The listing builds one solid part. Answer for the finished solid, in the listing's coordinates (mm). A direction names the side the tool comes from. Give positions to 0.01 mm unless a question says otherwise; leave off trailing zeros. Write each loop counter-clockwise with the first axis right and the second up, starting at its lowest first coordinate (ties: lowest second). Pieces come first, ordered by that corner, then holes. Notation, with made-up numbers: M 25.5,-5 L 72.5,-5 A18 ccw 72.5,21 Z; hole C 24,34 d1. An arc over 180 degrees is marked long. Answer as a JSON object with one key per item and string values.
```python
from build123d import *

# Parameters (mm, degrees)
SKETCH1_R           = 3.3274
BOSS_EXTRUDE1_DEPTH = 100


with BuildPart() as part:
    # Sketch1 → Boss-Extrude1 (new, symmetric)
    with BuildSketch(Plane.XY):
        with BuildLine():
            Line((-10.287, 13.552357131), (-10.287, 14.0843))
            ThreePointArc((-10.287, 14.0843), (-10.022898185, 14.721898185), (-9.3853, 14.986))
            Line((-9.3853, 14.986), (-5.617617549, 14.986))
            ThreePointArc((-5.617617549, 14.986), (-4.519044045, 15.441044045), (-4.064, 16.539617549))
            Line((-4.064, 16.539617549), (-4.064, 17.496382451))
            ThreePointArc((-4.064, 17.496382451), (-4.519044045, 18.594955955), (-5.617617549, 19.05))
            Line((-5.617617549, 19.05), (-7.974178704, 19.05))
            Line((-7.974178704, 19.05), (-15.847487039, 19.05))
            ThreePointArc((-15.847487039, 19.05), (-18.120176289, 18.120192083), (-19.05, 15.847509295))
            Line((-19.05, 15.847509295), (-19.05, 7.97632366))
            Line((-19.05, 7.97632366), (-19.05, 5.617617549))
            ThreePointArc((-19.05, 5.617617549), (-18.594955955, 4.519044045), (-17.496382451, 4.064))
            Line((-17.496382451, 4.064), (-16.539617549, 4.064))
            ThreePointArc((-16.539617549, 4.064), (-15.441044045, 4.519044045), (-14.986, 5.617617549))
            Line((-14.986, 5.617617549), (-14.986, 9.385342516))
            ThreePointArc((-14.986, 9.385342516), (-14.721898185, 10.022940701), (-14.0843, 10.287042516))
            Line((-14.0843, 10.287042516), (-13.516042086, 10.287042516))
            ThreePointArc((-13.516042086, 10.287042516), (-13.170975923, 10.218404478), (-12.878443117, 10.022939917))
            Line((-12.878443117, 10.022939917), (-8.14758008, 5.292065243))
            ThreePointArc((-8.14758008, 5.292065243), (-7.117955879, 3.751120653), (-6.7564, 1.933453584))
            Line((-6.7564, 1.933453584), (-6.7564, -1.933453584))
            ThreePointArc((-6.7564, -1.933453584), (-7.117955879, -3.751120653), (-8.14758008, -5.292065243))
            Line((-8.14758008, -5.292065243), (-12.878443117, -10.022939917))
            ThreePointArc((-12.878443117, -10.022939917), (-13.170975923, -10.218404478), (-13.516042086, -10.287042516))
            Line((-13.516042086, -10.287042516), (-14.0843, -10.287042516))
            ThreePointArc((-14.0843, -10.287042516), (-14.721898185, -10.022940701), (-14.986, -9.385342516))
            Line((-14.986, -9.385342516), (-14.986, -5.617617549))
            ThreePointArc((-14.986, -5.617617549), (-15.441044045, -4.519044045), (-16.539617549, -4.064))
            Line((-16.539617549, -4.064), (-17.496382451, -4.064))
            ThreePointArc((-17.496382451, -4.064), (-18.594955955, -4.519044045), (-19.05, -5.617617549))
            Line((-19.05, -5.617617549), (-19.05, -7.976318491))
            Line((-19.05, -7.976318491), (-19.05, -15.847510721))
            ThreePointArc((-19.05, -15.847510721), (-18.120175716, -18.120192644), (-15.847486868, -19.05))
            Line((-15.847486868, -19.05), (-7.976294616, -19.05))
            Line((-7.976294616, -19.05), (-5.617617549, -19.05))
            ThreePointArc((-5.617617549, -19.05), (-4.519044045, -18.594955955), (-4.064, -17.496382451))
            Line((-4.064, -17.496382451), (-4.064, -16.539617549))
            ThreePointArc((-4.064, -16.539617549), (-4.519044045, -15.441044045), (-5.617617549, -14.986))
            Line((-5.617617549, -14.986), (-9.3853, -14.986))
            ThreePointArc((-9.3853, -14.986), (-10.022898185, -14.721898185), (-10.287, -14.0843))
            Line((-10.287, -14.0843), (-10.287, -13.552357131))
            ThreePointArc((-10.287, -13.552357131), (-10.218362387, -13.207291992), (-10.022898969, -12.91475973))
            Line((-10.022898969, -12.91475973), (-5.252158105, -8.144007132))
            ThreePointArc((-5.252158105, -8.144007132), (-3.715177372, -7.117027388), (-1.902183975, -6.7564))
            Line((-1.902183975, -6.7564), (1.902183975, -6.7564))
            ThreePointArc((1.902183975, -6.7564), (3.715177372, -7.117027388), (5.252158105, -8.144007132))
            Line((5.252158105, -8.144007132), (10.022898969, -12.91475973))
            ThreePointArc((10.022898969, -12.91475973), (10.218362387, -13.207291992), (10.287, -13.552357131))
            Line((10.287, -13.552357131), (10.287, -14.0843))
            ThreePointArc((10.287, -14.0843), (10.022898185, -14.721898185), (9.3853, -14.986))
            Line((9.3853, -14.986), (5.617617549, -14.986))
            ThreePointArc((5.617617549, -14.986), (4.519044045, -15.441044045), (4.064, -16.539617549))
            Line((4.064, -16.539617549), (4.064, -17.496382451))
            ThreePointArc((4.064, -17.496382451), (4.519044045, -18.594955955), (5.617617549, -19.05))
            Line((5.617617549, -19.05), (7.976294616, -19.05))
            Line((7.976294616, -19.05), (15.847486868, -19.05))
            ThreePointArc((15.847486868, -19.05), (18.120175716, -18.120192644), (19.05, -15.847510721))
            Line((19.05, -15.847510721), (19.05, -7.976318491))
            Line((19.05, -7.976318491), (19.05, -5.617617549))
            ThreePointArc((19.05, -5.617617549), (18.594955955, -4.519044045), (17.496382451, -4.064))
            Line((17.496382451, -4.064), (16.539617549, -4.064))
            ThreePointArc((16.539617549, -4.064), (15.441044045, -4.519044045), (14.986, -5.617617549))
            Line((14.986, -5.617617549), (14.986, -9.385342516))
            ThreePointArc((14.986, -9.385342516), (14.721898185, -10.022940701), (14.0843, -10.287042516))
            Line((14.0843, -10.287042516), (13.516042086, -10.287042516))
            ThreePointArc((13.516042086, -10.287042516), (13.170975923, -10.218404478), (12.878443117, -10.022939917))
            Line((12.878443117, -10.022939917), (8.14758008, -5.292065243))
            ThreePointArc((8.14758008, -5.292065243), (7.117955879, -3.751120653), (6.7564, -1.933453584))
            Line((6.7564, -1.933453584), (6.7564, 1.933453584))
            ThreePointArc((6.7564, 1.933453584), (7.117955879, 3.751120653), (8.14758008, 5.292065243))
            Line((8.14758008, 5.292065243), (12.878443117, 10.022939917))
            ThreePointArc((12.878443117, 10.022939917), (13.170975923, 10.218404478), (13.516042086, 10.287042516))
            Line((13.516042086, 10.287042516), (14.0843, 10.287042516))
            ThreePointArc((14.0843, 10.287042516), (14.721898185, 10.022940701), (14.986, 9.385342516))
            Line((14.986, 9.385342516), (14.986, 5.617617549))
            ThreePointArc((14.986, 5.617617549), (15.441044045, 4.519044045), (16.539617549, 4.064))
            Line((16.539617549, 4.064), (17.496382451, 4.064))
            ThreePointArc((17.496382451, 4.064), (18.594955955, 4.519044045), (19.05, 5.617617549))
            Line((19.05, 5.617617549), (19.05, 9.496091471))
            Line((19.05, 9.496091471), (19.05, 15.847509295))
            ThreePointArc((19.05, 15.847509295), (18.120176289, 18.120192083), (15.847487039, 19.05))
            Line((15.847487039, 19.05), (7.974178704, 19.05))
            Line((7.974178704, 19.05), (5.617617549, 19.05))
            ThreePointArc((5.617617549, 19.05), (4.519044045, 18.594955955), (4.064, 17.496382451))
            Line((4.064, 17.496382451), (4.064, 16.539617549))
            ThreePointArc((4.064, 16.539617549), (4.519044045, 15.441044045), (5.617617549, 14.986))
            Line((5.617617549, 14.986), (9.3853, 14.986))
            ThreePointArc((9.3853, 14.986), (10.022898185, 14.721898185), (10.287, 14.0843))
            Line((10.287, 14.0843), (10.287, 13.552357131))
            ThreePointArc((10.287, 13.552357131), (10.218362387, 13.207291992), (10.022898969, 12.91475973))
            Line((10.022898969, 12.91475973), (5.252158105, 8.144007132))
            ThreePointArc((5.252158105, 8.144007132), (3.715177372, 7.117027388), (1.902183975, 6.7564))
            Line((1.902183975, 6.7564), (-1.902183975, 6.7564))
            ThreePointArc((-1.902183975, 6.7564), (-3.715177372, 7.117027388), (-5.252158105, 8.144007132))
            Line((-5.252158105, 8.144007132), (-10.022898969, 12.91475973))
            ThreePointArc((-10.022898969, 12.91475973), (-10.218362387, 13.207291992), (-10.287, 13.552357131))
        make_face()
        Circle(SKETCH1_R, mode=Mode.SUBTRACT)
    extrude(amount=BOSS_EXTRUDE1_DEPTH, both=True)


solid = part.part
```
1. A cutting plane is placed at A-A, the plane x = 0. Give the vertices of the cut face in (y, z), plus the area to 3 significant figures.
Verdict:
{"outline": "M -6.76,-100 L -3.33,-100 L -3.33,100 L -6.76,100 Z; M 3.33,-100 L 6.76,-100 L 6.76,100 L 3.33,100 Z", "area": "1,370 mm2"}
2. For faces 1 (the cylindrical face through (3.739, 7.127, 1.4)), 2 (the flat face through (6.756, 0, 1)), 3 (the flat face through (-6.756, 0, 1)), determine the directions among +Z, -Z, +X, -X, +Y, -Y from which every point of the face is accessible in a straight line to the end or side of a thin tool.
Verdict:
{"face 1": "+Z, -Z", "face 2": "+Z, -Z, +X", "face 3": "+Z, -Z, -X"}
3. Flat-ended cylindrical pins translate along their axes: pin 1 (0.8 mm diameter, centred on y = 17, z = 41.5, fed in from +X); pin 2 (1.5 mm diameter, centred on x = -2.5, z = -78.5, fed in from +Y); pin 3 (3 mm diameter, centred on y = -1, z = -18, fed in from +X). Find the tip coordinate at first contact, or state that the pin passes through.
Verdict:
{"pin 1": "stops at x = 18.97", "pin 2": "stops at y = 6.95", "pin 3": "stops at x = 6.79"}
4. The mould has two halves that part along X. Classify faces 4 (the flat face through (7.604, -10.496, 1.4)), 5 (the flat face through (19.05, 11, 1)), 6 (the cylindrical face through (7.13, -3.78, 1.4)), 7 (the flat face through (-5, 0, -100)): released by +X, released by -X, zero draft, split by the parting line, or undercut.
Verdict:
{"face 4": "undercut", "face 5": "released by +X", "face 6": "undercut", "face 7": "zero draft"}
5. Consider line 1 along Y through (x, z) = (-6.5, -78); line 2 along X through (y, z) = (6, 74); line 3 along Y through (x, z) = (0, -40). Determine where each line is inside the solid, lowest interval first.
Verdict:
{"line 1": "y = -19.05 to -14.99, -9.39 to 9.39, 14.99 to 19.05", "line 2": "x = -19.05 to -14.99, -8.86 to 8.86, 14.99 to 19.05", "line 3": "y = -6.76 to -3.33, 3.33 to 6.76"}
